Geometry check sheet. Reference: drawing and pictorial views, mm from the part's lowest x, y, z. Give positions to 0.01 mm unless a question says otherwise; leave off trailing zeros. Write each loop counter-clockwise with the first axis right and the second up, starting at its lowest first coordinate (ties: lowest second). Pieces come first, ordered by that corner, then holes. Notation, with made-up numbers: M 37,12.5 L 79,12.5 A23 ccw 79,25.5 Z; hole C 5.25,68.25 d4. An arc over 180 degrees is marked long. Answer as a JSON object with one key per item and string values.
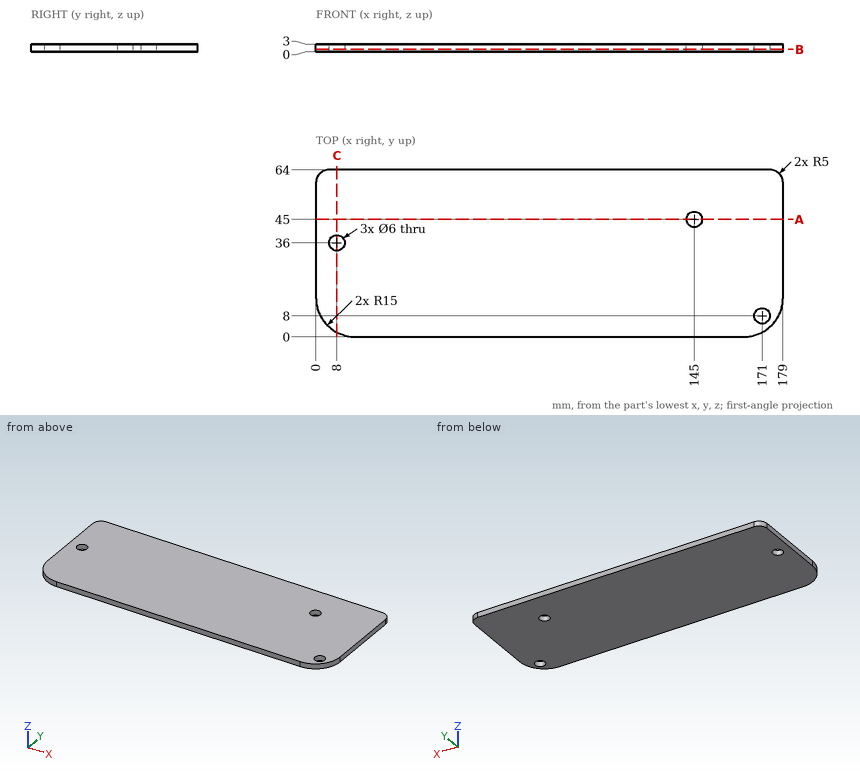
1) Section check C-C on x = 8. Record the boundary of the cut face in (y, z), and give its area (3 significant figures).
Completed:
{"outline": "M 1.73,0 L 33,0 L 33,3 L 1.73,3 Z; M 39,0 L 64,0 L 64,3 L 39,3 Z", "area": "169 mm2"}
2) Section check A-A on y = 45. Record the boundary of the cut face in (x, z).
Completed:
{"outline": "M 0,0 L 142,0 L 142,3 L 0,3 Z; M 148,0 L 179,0 L 179,3 L 148,3 Z"}
3) Section check B-B on z = 0.9. Record the boundary of the cut face in (x, y).
Completed:
{"outline": "M 0,15 A15 ccw 15,0 L 164,0 A15 ccw 179,15 L 179,59 A5 ccw 174,64 L 5,64 A5 ccw 0,59 Z; hole C 8,36 d6; hole C 145,45 d6; hole C 171,8 d6"}
4) Thickness scan on L1, parallel to Y at x = 145, z = 1.4; L2, parallel to X at y = 38, z = 2.15; L3, parallel to X at y = 47, z = 1.4. Record the ranges inside material, lowest first.
Completed:
{"L1": "y = 0 to 42, 48 to 64", "L2": "x = 0 to 5.76, 10.24 to 179", "L3": "x = 0 to 142.76, 147.24 to 179"}
5) Go/stop test with a flat-tipped pin: pin 1 (5 mm diameter, centred on x = 8, y = 36, fed in from +Z). Record where the tip stops, or that it passes through.
Completed:
{"pin 1": "passes through"}
